Could you check a few things on this model? Use its own coordinates, in mm. Round coordinates to 2 decimals unless told otherwise and drop trailing zeros. Loops run counter-clockwise (first coordinate to the right, second up) from the corner with the lowest first, then second, coordinate; pieces in that order, holes last. Notation, with made-up numbers: (86, 25.25) -> (123, 25.25) arc R22 cw to (123, 53.25) -> close; hole circle Ø8 at (20, 38.5). An arc over 180 degrees is marked (long way). Write each question's results on one line, items separated by ' | '.
from build123d import *

# Parameters (mm, degrees)
SKETCH_1_W             = 56
SKETCH_1_H             = 56
SM_BASE_FLANGE_1_DEPTH = 4
SKETCH_6_R             = 24.5
SKETCH_6_R_2           = 1.75
CUT_EXTRUDE_1_DEPTH    = 4
FILLET_1_R             = 3


# Sheet-metal steps are written as plain solids
with BuildPart() as part:
    # Sketch 1 → Базовая кромка1 (new body)
    with BuildSketch(Plane.XY):
        Rectangle(SKETCH_1_W, SKETCH_1_H)
    extrude(amount=-SM_BASE_FLANGE_1_DEPTH)

    # Эскиз6 → Вырез-Вытянуть1 (cut)
    with BuildSketch(Plane.XY):
        Circle(SKETCH_6_R)
        with Locations((-24, 24)):
            Circle(SKETCH_6_R_2)
        with Locations((24, 24)):
            Circle(SKETCH_6_R_2)
        with Locations((24, -24)):
            Circle(SKETCH_6_R_2)
        with Locations((-24, -24)):
            Circle(SKETCH_6_R_2)
    extrude(amount=-CUT_EXTRUDE_1_DEPTH, mode=Mode.SUBTRACT)

    # Скругление1
    fillet_1_edges = [part.edges().sort_by_distance(p)[0] for p in [
        (28, -28, -2),
        (-28, -28, -2),
        (-28, 28, -2),
        (28, 28, -2),
    ]]
    fillet(fillet_1_edges, radius=FILLET_1_R)


solid = part.part
1) I want a section at C-C, the plane z = -2.75. Write out the boundary of the cut face in (x, y).
Model answer:
outline: (-28, -25) arc R3 ccw to (-25, -28) -> (25, -28) arc R3 ccw to (28, -25) -> (28, 25) arc R3 ccw to (25, 28) -> (-25, 28) arc R3 ccw to (-28, 25) -> close; hole circle Ø3.5 at (-24, -24); hole circle Ø3.5 at (-24, 24); hole circle Ø49 at (0, 0); hole circle Ø3.5 at (24, -24); hole circle Ø3.5 at (24, 24)
2) If we mould it in two halves opening along Y, with no side actions, what happens to faces 1 (the flat face through (-25, 0, -4)), 2 (the cylindrical face through (-25.29, -22.82, -1.97)), 3 (the cylindrical face through (27.1, 27.14, -2.03)), 4 (the cylindrical face through (-25.29, 25.18, -1.97))? For each: released by +Y, released by -Y, zero draft, split by the parting line, or undercut.
Model answer:
face 1: zero draft | face 2: undercut | face 3: released by +Y | face 4: undercut
3) I want a section at A-A, the plane y = 0. Write out the boundary of the cut face in (x, z).
Model answer:
outline: (-28, -4) -> (-24.5, -4) -> (-24.5, 0) -> (-28, 0) -> close; (24.5, -4) -> (28, -4) -> (28, 0) -> (24.5, 0) -> close
4) I need wall thicknesses on line 1 (Y direction, x = 0, z = -2.25); line 2 (Y direction, x = -25, z = -3.1); line 3 (X direction, y = 18.5, z = -2.7). Which ranges of each line are inside material? Lowest first, please.
Model answer:
line 1: y = -28 to -24.5, 24.5 to 28 | line 2: y = -28 to -25.44, -22.56 to 22.56, 25.44 to 28 | line 3: x = -28 to -16.06, 16.06 to 28
5) I'm going to push a flat-ended pin straight in: pin 1 (2 mm diameter, centred on x = -24, y = 24, fed in from +Z). Where does the tip first touch, or does it pass through?
Model answer:
pin 1: passes through
